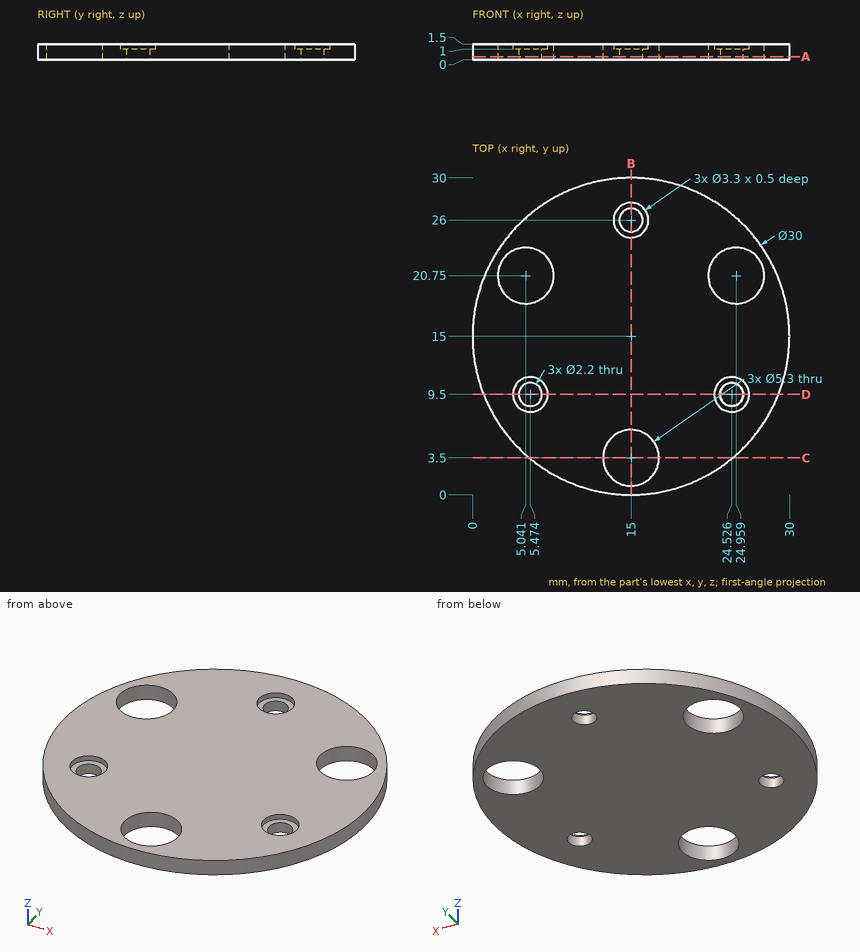
Answer from the drawing. Dimensions are ordinates in mm from the lowest x, y and z of the part. Coordinates: 2 decimals unless noted, no trailing zeros. Order: outer loops, then holes, each group sorted by start corner. A loop starts at its lowest first (then second) coordinate and runs counter-clockwise, first axis right, second up. Notation, with made-up numbers: (-24, -34.5) - (35, -34.5) arc R9 ccw to (35, -28.5) - close; hole circle Ø3 at (-6.5, 49.25). An arc over 180 degrees is marked (long way). Put each result on its own line as item: value. Start each with the question number.
1) A flat-ended cylindrical pin translates along its axis: pin 1 (3 mm diameter, centred on x = 5.47, y = 9.5, fed in from +Z). Find the tip coordinate at first contact, or state that the pin passes through.
2) Find section D-D (y = 9.5). Give the vertices of the cut face in (x, z) (1 decimal).
3) Find section C-C (y = 3.5). Give the vertices of the cut face in (x, z).
4) Find section A-A (z = 0.3). Give the vertices of the cut face in (x, y), plus the area to 3 significant figures.
5) Find the intervals of material crossed by line 1 (Y direction, x = 15, z = 1.45); line 2 (Y direction, x = 15, z = 0.5); line 3 (X direction, y = 19.25, z = 0.95) (1 decimal), in increasing order. Write a range as from..to.
6) Find section B-B (x = 15). Give the vertices of the cut face in (y, z).
Results list:
1. pin 1: stops at z = 1
2. outline: (1, 0) - (4.4, 0) - (4.4, 1) - (3.8, 1) - (3.8, 1.5) - (1, 1.5) - close; (6.6, 0) - (23.4, 0) - (23.4, 1) - (22.9, 1) - (22.9, 1.5) - (7.1, 1.5) - (7.1, 1) - (6.6, 1) - close; (25.6, 0) - (29, 0) - (29, 1.5) - (26.2, 1.5) - (26.2, 1) - (25.6, 1) - close
3. outline: (5.37, 0) - (12.35, 0) - (12.35, 1.5) - (5.37, 1.5) - close; (17.65, 0) - (24.63, 0) - (24.63, 1.5) - (17.65, 1.5) - close
4. outline: circle Ø30 at (15, 15); hole circle Ø5.3 at (5.04, 20.75); hole circle Ø2.2 at (5.47, 9.5); hole circle Ø5.3 at (15, 3.5); hole circle Ø2.2 at (15, 26); hole circle Ø5.3 at (24.96, 20.75); hole circle Ø2.2 at (24.53, 9.5)
4. area: 629 mm^2
5. line 1: y = 0..0.85, 6.15..24.35, 27.65..30
5. line 2: y = 0..0.85, 6.15..24.9, 27.1..30
5. line 3: x = 0.6..2.9, 7.2..22.8, 27.1..29.4
6. outline: (0, 0) - (0.85, 0) - (0.85, 1.5) - (0, 1.5) - close; (6.15, 0) - (24.9, 0) - (24.9, 1) - (24.35, 1) - (24.35, 1.5) - (6.15, 1.5) - close; (27.1, 0) - (30, 0) - (30, 1.5) - (27.65, 1.5) - (27.65, 1) - (27.1, 1) - close
